Geometry: final body of the model. Coordinates: model frame, mm. Face numbers are marked on the shaded views. A direction names the side the tool comes from. Give positions to 0.01 mm unless a question says otherwise; leave off trailing zeros. Loops run counter-clockwise (first coordinate to the right, second up) from the corner with the lowest first, then second, coordinate; pieces in that order, holes last.
```python
from build123d import *

# Parameters (mm, degrees)
F0_W      = 50
F0_H      = 50
F1_DEPTH  = 250
F3_R      = 4
F4_DEPTH  = 50.001
F5_W      = 6
F5_H      = 14
F5_W_2    = 14
F5_H_2    = 6
F6_DEPTH  = 250.001
F8_DEPTH  = 50.001
F9_R      = 10
F10_DEPTH = 35


with BuildPart() as f1:
    # F0 (on Front) → F1 (new body)
    with BuildSketch(Plane.XZ):
        Rectangle(F0_W, F0_H)
    extrude(amount=F1_DEPTH)

    # F3 (on face) → F4 (cut, through all)
    with BuildSketch(Plane(origin=(0, 0, -25), x_dir=(1, 0, 0), z_dir=(0, 0, -1))):
        with Locations((0, 825)):
            Circle(F3_R)
        with Locations((0, 625)):
            Circle(F3_R)
        with Locations((0, 425)):
            Circle(F3_R)
        with Locations((0, 225)):
            Circle(F3_R)
        with Locations((0, 25)):
            Circle(F3_R)
        with Locations((0, -175)):
            Circle(F3_R)
        with Locations((0, -375)):
            Circle(F3_R)
        with Locations((0, -575)):
            Circle(F3_R)
    extrude(amount=-F4_DEPTH, mode=Mode.SUBTRACT)

    # F5 (on face) → F6 (cut, through all)
    with BuildSketch(Plane.XZ.offset(250)):
        with Locations((0, 18)):
            Rectangle(F5_W, F5_H)
        with Locations((0, -18)):
            Rectangle(F5_W, F5_H)
        with Locations((-18, 50)):
            Rectangle(F5_W_2, F5_H_2)
        with Locations((-18, 0)):
            Rectangle(F5_W_2, F5_H_2)
        with Locations((-18, -50)):
            Rectangle(F5_W_2, F5_H_2)
        with Locations((18, 50)):
            Rectangle(F5_W_2, F5_H_2)
        with Locations((18, 0)):
            Rectangle(F5_W_2, F5_H_2)
        with Locations((18, -50)):
            Rectangle(F5_W_2, F5_H_2)
    extrude(amount=-F6_DEPTH, mode=Mode.SUBTRACT)

    # F7 (on face) → F8 (cut, through all)
    with BuildSketch(Plane(origin=(-25, 0, 0), x_dir=(0, -1, 0), z_dir=(-1, 0, 0))):
        Polygon((50, 25), (0, 25), (0, -25), align=None)
        Polygon((250, 25), (200, 25), (250, -25), align=None)
    extrude(amount=-F8_DEPTH, mode=Mode.SUBTRACT)

    # F9 (on face) → F10 (cut)
    with BuildSketch(Plane.YZ.offset(25)):
        with Locations((-197.5, 0)):
            Circle(F9_R)
        with Locations((-52.5, 0)):
            Circle(F9_R)
    extrude(amount=-F10_DEPTH, mode=Mode.SUBTRACT)


solid = f1.part
```
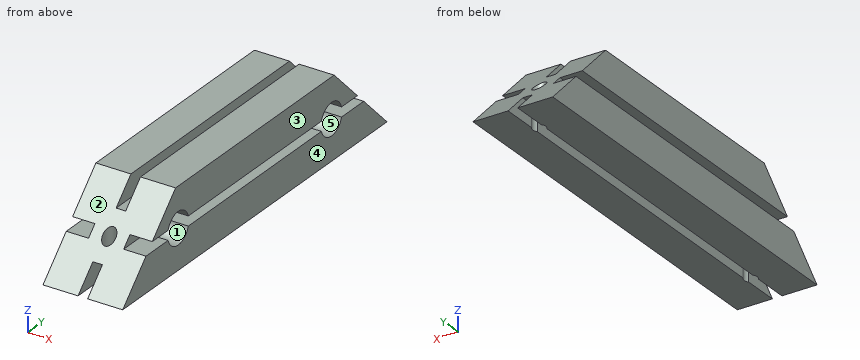
Q1. Pin query (flat end, axial travel): pin 1 Ø1 at (x, z) = (-11, -2) entering from +Y; pin 2 Ø5 at (x, z) = (-17, -3.5) entering from +Y; pin 3 Ø1.8 at (y, z) = (-220, 1.5) entering from +X; pin 4 Ø6.5 at (x, y) = (0.5, -142) entering from -Z. Return the tip coordinate at first contact, or that it passes through.
Q2. Section query C-C, the plane z = 20.5. Return loops of the section in (x, y), and give its area (3 significant figures).
Q3. Mould query, pull axis Z, two halves, no side actions, for the marked faces 1, 2 and 3. Classes: +Z half, -Z half, draft (parallel to the pull), parting line (faces both ways), or undercut.
Q4. Section query D-D, the plane x = -19.5. Return loops of the section in (y, z), and give its area (3 significant figures).
Q5. Reachability of the marked faces 4 and 5 from +Z, -Z, +X, -X, +Y, -Y: full face, straight path, thin tool, end or side. Return the list, or none.
Q6. Section query A-A, the plane x = 0. Return loops of the section in (y, z).
Q7. Material intervals for probe 1 along X at (y, z) = (-72, 18.5); probe 2 along Z at (x, y) = (-1, -52); probe 3 along Z at (x, y) = (-15, -35), sorted ascending.
Q8. Section query B-B, the plane y = -25. Return loops of the section in (x, z), and give its area (3 significant figures).
Resolved:
1. pin 1: stops at y = -22.5
1. pin 2: stops at y = -19
1. pin 3: stops at x = 11
1. pin 4: stops at z = -25
2. outline: (-25, -204.5) - (-3, -204.5) - (-3, -45.5) - (-25, -45.5) - close; (3, -204.5) - (25, -204.5) - (25, -45.5) - (3, -45.5) - close
2. area: 7,000 mm2
3. face 1: undercut
3. face 2: +Z half
3. face 3: draft
4. outline: (-250, -25) - (0, -25) - (-22, -3) - (-228, -3) - close; (-222, 3) - (-28, 3) - (-50, 25) - (-200, 25) - close
4. area: 8,800 mm2
5. face 4: +Z, -Z, +X, +Y, -Y
5. face 5: +X
6. outline: (-236, -11) - (-229, -11) - (-229, -4) - close; (-221, -11) - (-29, -11) - (-29, 4) - (-36, 11) - (-214, 11) - (-221, 4) - close; (-21, -11) - (-14, -11) - (-21, -4) - close; hole circle Ø20 at (-197.5, 0); hole circle Ø20 at (-52.5, 0)
7. probe 1: x = -25 to -3, 3 to 25
7. probe 2: z = -11 to -9.99, 9.99 to 11
7. probe 3: z = -25 to -3, 3 to 10
8. outline: (-25, -25) - (-4, -25) - (-4, 0) - (-11, 0) - (-11, -3) - (-25, -3) - close; (4, -25) - (25, -25) - (25, -3) - (11, -3) - (11, 0) - (4, 0) - close
8. area: 966 mm2
